```python
from build123d import *

# Parameters (mm, degrees)
SKETCH1_R           = 14.2875
SKETCH1_R_2         = 2.0193
BOSS_EXTRUDE1_DEPTH = 3.175
FILLET1_R           = 2.54
SKETCH2_R           = 14.2875
SKETCH2_R_2         = 2.6289
CUT_EXTRUDE1_DEPTH  = 238.443914509


with BuildPart() as part:
    # Sketch1 → Boss-Extrude1 (new body)
    with BuildSketch(Plane.XY):
        with BuildLine():
            Line((146.05, 146.96694), (-146.05, 164.23894))
            Line((-146.05, 164.23894), (-171.45, 164.23894))
            Line((-171.45, 164.23894), (-171.45, 113.43894))
            Line((-171.45, 113.43894), (-116.081416722, 103.131947821))
            ThreePointArc((-116.081416722, 103.131947821), (-90.681416722, 77.731947821), (-65.281416722, 103.131947821))
            Line((-65.281416722, 103.131947821), (100.376646224, 63.682232473))
            Line((100.376646224, 63.682232473), (111.82489431, 60.955953292))
            ThreePointArc((111.82489431, 60.955953292), (129.785406552, 68.395441049), (137.22489431, 86.355953292))
            Line((137.22489431, 86.355953292), (171.45, 96.16694))
            Line((171.45, 96.16694), (171.45, 146.96694))
            Line((171.45, 146.96694), (146.05, 146.96694))
        make_face()
        with Locations((-90.681416722, 103.131947821)):
            Circle(SKETCH1_R, mode=Mode.SUBTRACT)
        with Locations((111.82489431, 86.355953292)):
            Circle(SKETCH1_R, mode=Mode.SUBTRACT)
        with Locations((158.75, 108.86694)):
            Circle(SKETCH1_R_2, mode=Mode.SUBTRACT)
        with Locations((-158.75, 126.13894)):
            Circle(SKETCH1_R_2, mode=Mode.SUBTRACT)
        with Locations((-158.75, 151.53894)):
            Circle(SKETCH1_R_2, mode=Mode.SUBTRACT)
        with Locations((158.75, 134.26694)):
            Circle(SKETCH1_R_2, mode=Mode.SUBTRACT)
    extrude(amount=BOSS_EXTRUDE1_DEPTH)

    # Fillet1
    # the kernel refuses this fillet: 2.54 mm, written as the material it adds along each edge
    with BuildSketch(Plane(origin=(-116.081416722, 103.131947821, 0), x_dir=(0.03807134416902504, -0.9992750235811778, 0), z_dir=(0, 0, 1))) as fillet1_piece_1:
        with BuildLine():
            CenterArc((2.030725498, -2.53815856), FILLET1_R, 92.181854631, 75.091245619)
            Line((-0.446869803, -1.978585935), (0, 0))
            ThreePointArc((0, 0), (0.967012142, -0.018414401), (1.934024284, 0))
        make_face()
    extrude(amount=3.175)
    with BuildSketch(Plane(origin=(146.05, 146.96694, 0), x_dir=(-0.9982563668513765, 0.05902733299658733, 0), z_dir=(0, 0, 1))) as fillet1_piece_2:
        with BuildLine():
            CenterArc((FILLET1_R * 0.0295394194538, -FILLET1_R), FILLET1_R, 90, 3.383984094)
            Line((-FILLET1_R * 0.0294879135427, -FILLET1_R * 0.00174363314863), (0, 0))
            Line((0, 0), (FILLET1_R * 0.0295394194537, 0))
        make_face()
    extrude(amount=3.175)
    with BuildSketch(Plane(origin=(137.22489431, 86.355953292, 0), x_dir=(0.9612833075503745, 0.2755619760144931, 0), z_dir=(0, 0, 1))) as fillet1_piece_3:
        with BuildLine():
            CenterArc((1.844513026, -2.54), FILLET1_R, 90, 70.036589556)
            ThreePointArc((-0.542860523, -1.672793255), (-0.256948075, -0.841096436), (0, 0))
            Line((0, 0), (1.844513026, 0))
        make_face()
    extrude(amount=3.175)
    # the kernel refuses this fillet: 2.54 mm, written as the material it takes off along each edge
    with BuildSketch(Plane(origin=(-171.45, 113.43894, -5.277017888), x_dir=(0, 1, 0), z_dir=(0, 0, 1))) as fillet1_2_piece_1:
        with BuildLine():
            CenterArc((FILLET1_R * 0.831026439026, -FILLET1_R), FILLET1_R, 90, 79.454954882)
            Line((-FILLET1_R * 0.152084893732, -FILLET1_R * 0.816991510029), (0, 0))
            Line((0, 0), (FILLET1_R * 0.831026439026, 0))
        make_face()
    extrude(amount=13.729035776, mode=Mode.SUBTRACT)
    with BuildSketch(Plane(origin=(-171.45, 164.23894, -6.35), x_dir=(1, 0, 0), z_dir=(0, 0, 1)), Plane(origin=(171.45, 146.96694, -6.35), x_dir=(0, -1, 0), z_dir=(0, 0, 1))) as fillet1_2_piece_2:
        with BuildLine():
            CenterArc((FILLET1_R, -FILLET1_R), FILLET1_R, 90, 90)
            Line((0, -FILLET1_R), (0, 0))
            Line((0, 0), (FILLET1_R, 0))
        make_face()
    extrude(amount=15.875, mode=Mode.SUBTRACT)
    with BuildSketch(Plane(origin=(171.45, 96.16694, -4.78545858), x_dir=(-0.9612833075503753, -0.2755619760144905, 0), z_dir=(0, 0, 1))) as fillet1_2_piece_3:
        with BuildLine():
            CenterArc((FILLET1_R * 0.753615524472, -FILLET1_R), FILLET1_R, 90, 74.004492945)
            Line((-FILLET1_R * 0.207667783079, -FILLET1_R * 0.724438023986), (0, 0))
            Line((0, 0), (FILLET1_R * 0.753615524472, 0))
        make_face()
    extrude(amount=12.745917161, mode=Mode.SUBTRACT)

    # Sketch2 → Cut-Extrude1 (cut, through all)
    with BuildSketch(Plane.XY.offset(3.175)):
        with Locations((76.380709582, 115.23549915)):
            Circle(SKETCH2_R)
        with Locations((76.380709582, 140.63549915)):
            Circle(SKETCH2_R_2)
        with Locations((101.780709582, 115.23549915)):
            Circle(SKETCH2_R_2)
        with Locations((76.380709582, 89.83549915)):
            Circle(SKETCH2_R_2)
        with Locations((50.980709582, 115.23549915)):
            Circle(SKETCH2_R_2)
    extrude(amount=-CUT_EXTRUDE1_DEPTH, mode=Mode.SUBTRACT)


solid = part.part
```
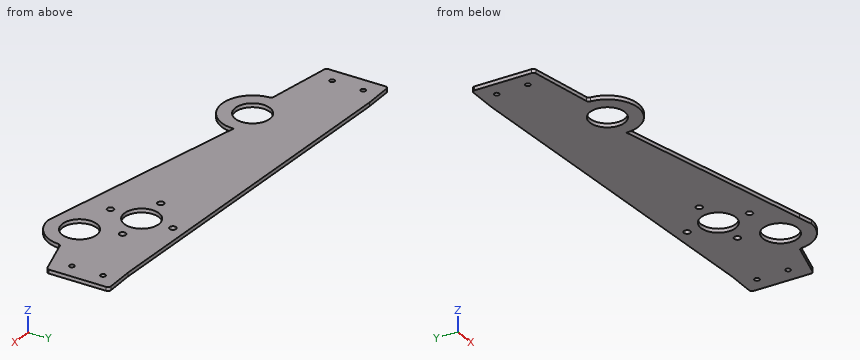
For this review, take the finished solid that the model builds, in its own axes (mm). Round coordinates to 2 decimals unless told otherwise and drop trailing zeros. Write each loop counter-clockwise with the first axis right and the second up, starting at its lowest first coordinate (ties: lowest second). Pieces come first, ordered by that corner, then holes. Notation, with made-up numbers: (1, 5.25) - (54, 5.25) arc R9 ccw to (54, 12.25) - close; hole circle Ø1 at (56, 82). An arc over 180 degrees is marked (long way). Answer as a JSON object with one key per item and string values.
1. To check wall thickness, follow line 1 along Y through (x, z) = (-158.75, 1.65); line 2 along X through (y, z) = (113.5, 0.55); line 3 along X through (y, z) = (117.5, 0.55). State the ranges of each line that lie inside material, in increasing order.
Response values:
{"line 1": "y = 111.07 to 124.12, 128.16 to 149.52, 153.56 to 164.24", "line 2": "x = -170.41 to -100.51, -80.85 to 49.01, 52.96 to 62.2, 90.56 to 99.81, 103.76 to 171.45", "line 3": "x = -171.45 to 49.65, 52.32 to 62.27, 90.49 to 100.45, 103.12 to 171.45"}
2. We need section C-C on x = 41. Give the boundary of the cut face in (y, z) (3 decimals).
Response values:
{"outline": "(77.822, 0) - (153.179, 0) - (153.179, 3.175) - (77.822, 3.175) - close"}
3. We need section B-B on z = 1.5. Count the separate pieces of the cut face and the enclosed holes in it, then the cut area to 3 significant figures.
Response values:
{"separate pieces": "1", "enclosed holes": "11", "area": "21,700 mm2"}
4. We need section A-A on x = -100. Give the boundary of the cut face in (y, z) (3 decimals), then the cut area to 3 significant figures.
Response values:
{"outline": "(79.503, 0) - (92.302, 0) - (92.302, 3.175) - (79.503, 3.175) - close; (113.962, 0) - (161.516, 0) - (161.516, 3.175) - (113.962, 3.175) - close", "area": "192 mm2"}
